```python
from build123d import *

# Parameters (mm, degrees)
BOSS_EXTRU_1_DEPTH       = 5
BOSS_EXTRU_1_DEPTH_BACK  = 5
ENL_V_MAT_EXTRU_10_DEPTH = 231.054341407
ENL_V_MAT_EXTRU_11_DEPTH = 228.935297837
CONG_1_R                 = 5
ESQUISSE16_R             = 1.5
ENL_V_MAT_EXTRU_13_DEPTH = 218.86334593
ESQUISSE17_R             = 1.5
ENL_V_MAT_EXTRU_14_DEPTH = 122.257222097
ENL_V_START              = -3
ENL_V_MAT_EXTRU_15_DEPTH = 119.257222101
ENL_V_MAT_EXTRU_16_DEPTH = 164.547347768
CONG_2_R                 = 1


with BuildPart() as part:
    # Esquisse1 → Boss.-Extru.1 (new, two sides: drawn at the far end of the back side and taken through both)
    with BuildSketch(Plane(origin=(0, 0, 0), x_dir=(1, 0, 0), z_dir=(0, 1, 0)).offset(-BOSS_EXTRU_1_DEPTH_BACK)):
        with BuildLine():
            Line((0, 49), (165, 49))
            Line((165, 49), (165, -55.235857919))
            ThreePointArc((165, -55.235857919), (127.908511428, -117.963607542), (68.381283989, -160))
            Line((68.381283989, -160), (0, -160))
            Line((0, -160), (0, 49))
        make_face()
    extrude(amount=BOSS_EXTRU_1_DEPTH + BOSS_EXTRU_1_DEPTH_BACK)

    # Sym_trie1: part across plane


with BuildPart() as part_1:
    add(part.part)
    add(part.part.mirror(Plane(origin=(0, -5, -49), x_dir=(0, 0, 1), z_dir=(-1, 0, 0))))

    # Esquisse12 → Enl_v. mat.-Extru.10 (cut, through all)
    with BuildSketch(Plane(origin=(0, 5, 0), x_dir=(1, 0, 0), z_dir=(0, 1, 0))):
        with BuildLine():
            Line((165, 49), (-165, 49))
            Line((-165, 49), (-165, -55.235857919))
            ThreePointArc((-165, -55.235857919), (-127.908511428, -117.963607542), (-68.381283989, -160))
            Line((-68.381283989, -160), (68.381283989, -160))
            ThreePointArc((68.381283989, -160), (127.908511428, -117.963607542), (165, -55.235857919))
            Line((165, -55.235857919), (165, 49))
        make_face()
        with BuildLine():
            Line((163.5, 47.5), (-163.5, 47.5))
            Line((-163.5, 47.5), (-163.5, -54.990908339))
            ThreePointArc((-163.5, -54.990908339), (-126.827060587, -116.923678966), (-68.0734897, -158.5))
            Line((-68.0734897, -158.5), (68.0734897, -158.5))
            ThreePointArc((68.0734897, -158.5), (126.827060587, -116.923678966), (163.5, -54.990908339))
            Line((163.5, -54.990908339), (163.5, 47.5))
        make_face(mode=Mode.SUBTRACT)
    extrude(amount=-ENL_V_MAT_EXTRU_10_DEPTH, mode=Mode.SUBTRACT)

    # Esquisse13 → Enl_v. mat.-Extru.11 (cut, through all)
    with BuildSketch(Plane(origin=(0, 5, 0), x_dir=(1, 0, 0), z_dir=(0, 1, 0))):
        with BuildLine():
            Line((-163.5, 47.5), (163.5, 47.5))
            Line((163.5, 47.5), (163.5, -158.5))
            Line((163.5, -158.5), (0, -158.5))
            Line((0, -158.5), (0, -152.5))
            Line((0, -152.5), (-66.828137786, -152.5))
            ThreePointArc((-66.828137786, -152.5), (-111.046814507, -124.059884684), (-144.19322973, -83.25))
            Line((-144.19322973, -83.25), (-163.5, -94.396769013))
            Line((-163.5, -94.396769013), (-163.5, 47.5))
        make_face()
    extrude(amount=-ENL_V_MAT_EXTRU_11_DEPTH, mode=Mode.SUBTRACT)

    # Cong_1
    cong_1_edges = [part_1.edges().sort_by_distance(p)[0] for p in [
        (-68.0734897, 0, 158.5),
        (-144.19322973, 0, 83.25),
    ]]
    fillet(cong_1_edges, radius=CONG_1_R)

    # Esquisse16 → Enl_v. mat.-Extru.13 (cut, through all)
    with BuildSketch(Plane.XY):
        with Locations((-50, 0)):
            Circle(ESQUISSE16_R)
    extrude(amount=ENL_V_MAT_EXTRU_13_DEPTH, mode=Mode.SUBTRACT)

    # Esquisse17 → Enl_v. mat.-Extru.14 (cut, through all)
    with BuildSketch(Plane(origin=(-112.029788337, 0, 131.170029066), x_dir=(0, 1, 0), z_dir=(-0.6494480483301822, 0, 0.7604059656000322))):
        with Locations(Location((0, 0, 0), (0, 0, 270))):
            Circle(ESQUISSE17_R)
    extrude(amount=-ENL_V_MAT_EXTRU_14_DEPTH, mode=Mode.SUBTRACT)

    # Esquisse18 → Enl_v. mat.-Extru.15 (cut, through all)
    with BuildSketch(Plane(origin=(-112.029788337, 0, 131.170029066), x_dir=(0, 1, 0), z_dir=(-0.6494480483301822, 0, 0.7604059656000322)).offset(ENL_V_START)):
        Polygon((3.175426481, 0), (1.58771324, 2.75), (-1.58771324, 2.75), (-3.175426481, 0), (-1.58771324, -2.75), (1.58771324, -2.75), align=None)
    extrude(amount=-ENL_V_MAT_EXTRU_15_DEPTH, mode=Mode.SUBTRACT)

    # Esquisse19 → Enl_v. mat.-Extru.16 (cut, through all)
    with BuildSketch(Plane.XY.offset(158.5).offset(ENL_V_START)):
        Polygon((-47.25, -1.58771324), (-47.25, 1.58771324), (-50, 3.175426481), (-52.75, 1.58771324), (-52.75, -1.58771324), (-50, -3.175426481), align=None)
    extrude(amount=-ENL_V_MAT_EXTRU_16_DEPTH, mode=Mode.SUBTRACT)

    # Cong_2
    cong_2_edges = [part_1.edges().sort_by_distance(p)[0] for p in [
        (-109.226367496, 5, 125.665630319),
        (-109.226367496, -5, 125.665630319),
        (-144.736674491, 5, 85.195693901),
        (-144.736674491, -5, 85.195693901),
        (-148.924802049, -5, 85.981774552),
        (-33.414068893, -5, 152.5),
        (-148.924802049, 5, 85.981774552),
        (-33.414068893, 5, 152.5),
    ]]
    fillet(cong_2_edges, radius=CONG_2_R)

    # Sym_trie2: part across plane


with BuildPart() as part_2:
    add(part_1.part)
    add(part_1.part.mirror(Plane(origin=(0, -5, 152.5), x_dir=(0, 0, 1), z_dir=(-1, 0, 0))))


solid = part_2.part
```
Model file for the job. Use its own axes, mm. A direction names the side the tool comes from. Give positions to 0.01 mm unless a question says otherwise; leave off trailing zeros. Order: outer loops, then holes, each group sorted by start corner. A loop starts at its lowest first (then second) coordinate and runs counter-clockwise, first axis right, second up.
1) Wall check: probe 1 along Y at (x, z) = (50, 157); probe 2 along X at (y, z) = (0, 157); probe 3 along X at (y, z) = (0, 157.5). Give the ranges that are in metal, low to high.
2) Pin check, flat tips, straight feed: pin 1 (0.9 mm diameter, centred on y = 0, z = 154, fed in from -X); pin 2 (5 mm diameter, centred on y = 1, z = 125.5, fed in from -X); pin 3 (1 mm diameter, centred on y = 3.5, z = 119.5, fed in from +X); pin 4 (1.8 mm diameter, centred on x = 50, y = 0, fed in from -Z). Stop position of each tip, or through.
3) 3-axis set-ups, long thin cutter, end or side, ignore diameter. For faces 1 (the cylindrical face through (108.69, -3.5, 126.13)), 2 (the flat face through (1, 5, 154)), 3 (the flat face through (-51.3, -1.4, 155.5)): which of +Z, -Z, +X, -X, +Y, -Y reach the whole face in a straight line?
4) Saw through at A-A, the plane x = 19. Write the cut outline in (y, z).
5) Mould opens along Y. For faces 4 (the flat face through (-1, 0, 152.5)), 5 (the flat face through (51.3, -1.4, 155.5)), 6 (the flat face through (1, -5, 154)) say: +Y half, -Y half, draft (parallel to the pull), parting line (faces both ways), or undercut.
Computed:
1. probe 1: y = -5 to -1.5, 1.5 to 5
1. probe 2: x = -71.47 to -51.5, -48.5 to 48.5, 51.5 to 71.47
1. probe 3: x = -70.36 to -51.5, -48.5 to 48.5, 51.5 to 70.36
2. pin 1: stops at x = -78.6
2. pin 2: stops at x = -120.94
2. pin 3: stops at x = 124.88
2. pin 4: passes through
3. face 1: -Z, +Y, -Y
3. face 2: +Z, -Z, +X, -X, +Y
3. face 3: -Z
4. outline: (-5, 153.5) arc R1 ccw to (-4, 152.5) - (4, 152.5) arc R1 ccw to (5, 153.5) - (5, 158.5) - (-5, 158.5) - close
5. face 4: draft
5. face 5: undercut
5. face 6: -Y half
